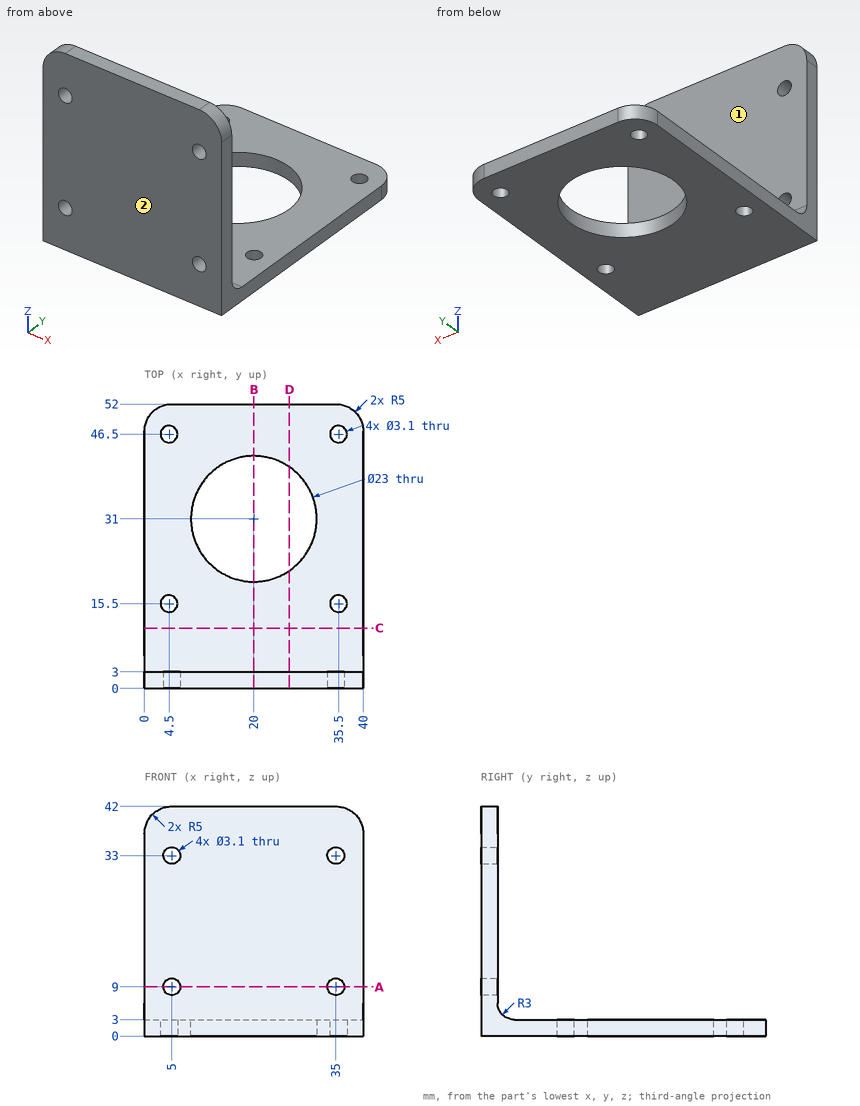
Can you work these out from the drawing? Everything is in mm from the part's minimum corner. A direction names the side the tool comes from. Give positions to 0.01 mm unless a question says otherwise; leave off trailing zeros. Write each loop counter-clockwise with the first axis right and the second up, starting at its lowest first coordinate (ties: lowest second). Pieces come first, ordered by that corner, then holes. Notation, with made-up numbers: (38, 10.25) -> (60, 10.25) arc R24 ccw to (60, 41.25) -> close; hole circle Ø5 at (51, 41.5). An arc over 180 degrees is marked (long way). Write each question's results on one line, items separated by ' | '.
Item 1: Suppose I cut it at A-A on z = 9. Write out the boundary of the cut face in (x, y), plus the area to 3 significant figures.
Output:
outline: (0, 0) -> (3.45, 0) -> (3.45, 3) -> (0, 3) -> close; (6.55, 0) -> (33.45, 0) -> (33.45, 3) -> (6.55, 3) -> close; (36.55, 0) -> (40, 0) -> (40, 3) -> (36.55, 3) -> close | area: 101 mm^2
Item 2: If I drill on L1, parallel to X at y = 0.7, z = 33; L2, parallel to Y at x = 20, z = 1; L3, parallel to Y at x = 35.5, z = 2.25, over which ranges is the centre line in solid material (lowest first)?
Output:
L1: x = 0 to 3.45, 6.55 to 33.45, 36.55 to 40 | L2: y = 0 to 19.5, 42.5 to 52 | L3: y = 0 to 13.95, 17.05 to 44.95, 48.05 to 51.97
Item 3: Suppose I cut it at B-B on x = 20. Write out the boundary of the cut face in (y, z), plus the area to 3 significant figures.
Output:
outline: (0, 0) -> (19.5, 0) -> (19.5, 3) -> (6, 3) arc R3 cw to (3, 6) -> (3, 42) -> (0, 42) -> close; (42.5, 0) -> (52, 0) -> (52, 3) -> (42.5, 3) -> close | area: 206 mm^2
Item 4: On a 3-axis mill with a long thin cutter (end or side, diameter ignored), from which of +Z, -Z, +X, -X, +Y, -Y can I reach the whole of each face in a straight line? I mean the marked faces 1 and 2. Say none if no direction works.
Output:
face 1: +Z, +X, -X, +Y | face 2: +Z, -Z, +X, -X, -Y
Item 5: For pin 1 Ø11 at (x, z) = (28, 28.5) entering from +Y; pin 2 Ø2 at (x, y) = (8.5, 41) entering from +Z, each with a flat end and sliding along its axis, tell me the tip position at first contact or that it passes through.
Output:
pin 1: stops at y = 3 | pin 2: stops at z = 3
Item 6: Suppose I cut it at D-D on x = 26.5. Write out the boundary of the cut face in (y, z), plus the area to 3 significant figures.
Output:
outline: (0, 0) -> (21.51, 0) -> (21.51, 3) -> (6, 3) arc R3 cw to (3, 6) -> (3, 42) -> (0, 42) -> close; (40.49, 0) -> (52, 0) -> (52, 3) -> (40.49, 3) -> close | area: 218 mm^2
Item 7: Suppose I cut it at C-C on y = 11. Write out the boundary of the cut face in (x, z).
Output:
outline: (0, 0) -> (40, 0) -> (40, 3) -> (0, 3) -> close
